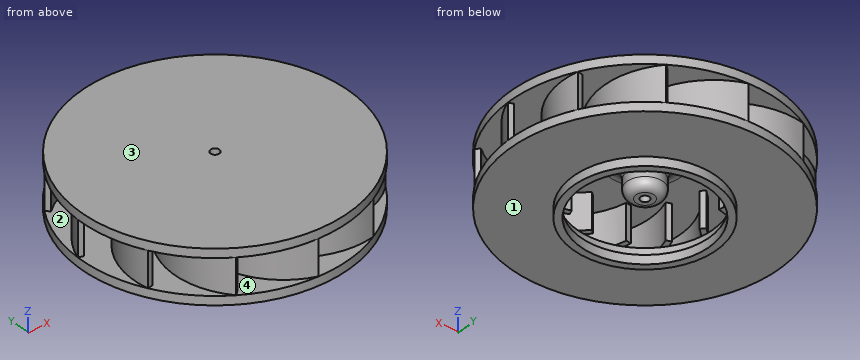
```python
from build123d import *

# Parameters (mm, degrees)
SKETCH_1_R          = 15
EXTRUDE_1_DEPTH     = 1
EXTRUDE_4_DEPTH     = 5
SKETCH_3_R          = 2
EXTRUDE_2_DEPTH     = 4
FILLET_1_R          = 2
FILLET_2_R          = 1
SKETCH_4_R          = 0.5
CUT_EXTRUDE_1_DEPTH = 5
SKETCH_5_R          = 15
EXTRUDE_3_DEPTH     = 1
SKETCH_6_R          = 8
SKETCH_6_R_2        = 7.2
EXTRUDE_4_2_DEPTH   = 1
SKETCH_7_R          = 7.6
CUT_EXTRUDE_2_DEPTH = 1


with BuildPart() as part:
    # 草图1 → 凸台-拉伸1 (new body)
    with BuildSketch(Plane.XY):
        Circle(SKETCH_1_R)
    extrude(amount=EXTRUDE_1_DEPTH)

    # 草图2 → Extrude 4 (add)
    with BuildSketch(Plane(origin=(0, 0, 0), x_dir=(-1, 0, 0), z_dir=(0, 0, -1))):
        with BuildLine():
            ThreePointArc((0, 7), (6.025450773, 10.246079868), (12.557822256, 8.203724775))
            Line((12.557822256, 8.203724775), (12.170554132, 7.745441675))
            ThreePointArc((12.170554132, 7.745441675), (6.082701111, 9.648817447), (0.467273577, 6.623628635))
            Line((0.467273577, 6.623628635), (0, 7))
        make_face()
        with BuildLine():
            ThreePointArc((3.5, 6.062177826), (10.341233372, 5.860640068), (14.977255477, 0.825722933))
            Line((14.977255477, 0.825722933), (14.412729894, 0.622472188))
            ThreePointArc((14.412729894, 0.622472188), (10.092182409, 5.31477047), (3.716485105, 5.502593875))
            Line((3.716485105, 5.502593875), (3.5, 6.062177826))
        make_face()
        with BuildLine():
            ThreePointArc((6.062177826, 3.5), (11.886090841, -0.095153505), (13.383545189, -6.773530702))
            Line((13.383545189, -6.773530702), (12.79302632, -6.667288219))
            ThreePointArc((12.79302632, -6.667288219), (11.397471581, -0.443364962), (5.969867451, 2.907143529))
            Line((5.969867451, 2.907143529), (6.062177826, 3.5))
        make_face()
        with BuildLine():
            ThreePointArc((7, 0), (10.246079868, -6.025450773), (8.203724775, -12.557822256))
            Line((8.203724775, -12.557822256), (7.745441675, -12.170554132))
            ThreePointArc((7.745441675, -12.170554132), (9.648817447, -6.082701111), (6.623628635, -0.467273577))
            Line((6.623628635, -0.467273577), (7, 0))
        make_face()
        with BuildLine():
            ThreePointArc((6.062177826, -3.5), (5.860640068, -10.341233372), (0.825722933, -14.977255477))
            Line((0.825722933, -14.977255477), (0.622472188, -14.412729894))
            ThreePointArc((0.622472188, -14.412729894), (5.31477047, -10.092182409), (5.502593875, -3.716485105))
            Line((5.502593875, -3.716485105), (6.062177826, -3.5))
        make_face()
        with BuildLine():
            ThreePointArc((3.5, -6.062177826), (-0.095153505, -11.886090841), (-6.773530702, -13.383545189))
            Line((-6.773530702, -13.383545189), (-6.667288219, -12.79302632))
            ThreePointArc((-6.667288219, -12.79302632), (-0.443364962, -11.397471581), (2.907143529, -5.969867451))
            Line((2.907143529, -5.969867451), (3.5, -6.062177826))
        make_face()
        with BuildLine():
            ThreePointArc((0, -7), (-6.025450773, -10.246079868), (-12.557822256, -8.203724775))
            Line((-12.557822256, -8.203724775), (-12.170554132, -7.745441675))
            ThreePointArc((-12.170554132, -7.745441675), (-6.082701111, -9.648817447), (-0.467273577, -6.623628635))
            Line((-0.467273577, -6.623628635), (0, -7))
        make_face()
        with BuildLine():
            ThreePointArc((-3.5, -6.062177826), (-10.341233372, -5.860640068), (-14.977255477, -0.825722933))
            Line((-14.977255477, -0.825722933), (-14.412729894, -0.622472188))
            ThreePointArc((-14.412729894, -0.622472188), (-10.092182409, -5.31477047), (-3.716485105, -5.502593875))
            Line((-3.716485105, -5.502593875), (-3.5, -6.062177826))
        make_face()
        with BuildLine():
            ThreePointArc((-6.062177826, -3.5), (-11.886090841, 0.095153505), (-13.383545189, 6.773530702))
            Line((-13.383545189, 6.773530702), (-12.79302632, 6.667288219))
            ThreePointArc((-12.79302632, 6.667288219), (-11.397471581, 0.443364962), (-5.969867451, -2.907143529))
            Line((-5.969867451, -2.907143529), (-6.062177826, -3.5))
        make_face()
        with BuildLine():
            ThreePointArc((-7, 0), (-10.246079868, 6.025450773), (-8.203724775, 12.557822256))
            Line((-8.203724775, 12.557822256), (-7.745441675, 12.170554132))
            ThreePointArc((-7.745441675, 12.170554132), (-9.648817447, 6.082701111), (-6.623628635, 0.467273577))
            Line((-6.623628635, 0.467273577), (-7, 0))
        make_face()
        with BuildLine():
            ThreePointArc((-6.062177826, 3.5), (-5.860640068, 10.341233372), (-0.825722933, 14.977255477))
            Line((-0.825722933, 14.977255477), (-0.622472188, 14.412729894))
            ThreePointArc((-0.622472188, 14.412729894), (-5.31477047, 10.092182409), (-5.502593875, 3.716485105))
            Line((-5.502593875, 3.716485105), (-6.062177826, 3.5))
        make_face()
        with BuildLine():
            ThreePointArc((-3.5, 6.062177826), (0.095153505, 11.886090841), (6.773530702, 13.383545189))
            Line((6.773530702, 13.383545189), (6.667288219, 12.79302632))
            ThreePointArc((6.667288219, 12.79302632), (0.443364962, 11.397471581), (-2.907143529, 5.969867451))
            Line((-2.907143529, 5.969867451), (-3.5, 6.062177826))
        make_face()
    extrude(amount=EXTRUDE_4_DEPTH)

    # 草图3 → 凸台-拉伸2 (add)
    with BuildSketch(Plane(origin=(0, 0, 0), x_dir=(-1, 0, 0), z_dir=(0, 0, -1))):
        with Locations(Location((0, 0, 0), (0, 0, 180))):
            Circle(SKETCH_3_R)
    extrude(amount=EXTRUDE_2_DEPTH)

    # 圆角1
    fillet_1_edges = [part.edges().sort_by_distance(p)[0] for p in [
        (-2, 0, 0),
    ]]
    fillet(fillet_1_edges, radius=FILLET_1_R)

    # 圆角2
    fillet_2_edges = [part.edges().sort_by_distance(p)[0] for p in [
        (-2, 0, -4),
    ]]
    fillet(fillet_2_edges, radius=FILLET_2_R)

    # 草图4 → 切除-拉伸1 (cut)
    with BuildSketch(Plane.XY.offset(1)):
        Circle(SKETCH_4_R)
    extrude(amount=-CUT_EXTRUDE_1_DEPTH, mode=Mode.SUBTRACT)

    # 草图5 → 凸台-拉伸3 (add)
    with BuildSketch(Plane(origin=(0, 0, -5), x_dir=(-1, 0, 0), z_dir=(0, 0, -1))):
        with Locations(Location((0, 0, 0), (0, 0, 3.155624395))):
            Circle(SKETCH_5_R)
    extrude(amount=-EXTRUDE_3_DEPTH)

    # 草图6 → Extrude 4 2 (add)
    with BuildSketch(Plane(origin=(0, 0, -5), x_dir=(-1, 0, 0), z_dir=(0, 0, -1))):
        Circle(SKETCH_6_R)
        Circle(SKETCH_6_R_2, mode=Mode.SUBTRACT)
    extrude(amount=EXTRUDE_4_2_DEPTH)

    # 草图7 → 切除-拉伸2 (cut)
    with BuildSketch(Plane(origin=(0, 0, -5), x_dir=(-1, 0, 0), z_dir=(0, 0, -1))):
        Circle(SKETCH_7_R)
    extrude(amount=-CUT_EXTRUDE_2_DEPTH, mode=Mode.SUBTRACT)


solid = part.part
```
Source: CAD feature listing. Evaluate the final solid. Frame: model axes, mm. Face numbers are marked on the shaded views. A direction names the side the tool comes from. Coordinates: 2 decimals unless noted, no trailing zeros. Order: outer loops, then holes, each group sorted by start corner. A loop starts at its lowest first (then second) coordinate and runs counter-clockwise, first axis right, second up. Notation, with made-up numbers: (83.5, 89.25) - (118.5, 89.25) arc R8 ccw to (118.5, 98.25) - close; hole circle Ø1 at (-0.75, 3). An arc over 180 degrees is marked (long way). One line per item, written item: value.
1) Cut plane A-A on y = -8.75. Output: boundary loops of the cut face in (x, z), plus the area to 3 significant figures.
Computed values:
outline: (-12.18, -5) - (12.18, -5) - (12.18, -4) - (11.84, -4) - (11.84, 0) - (12.18, 0) - (12.18, 1) - (-12.18, 1) - (-12.18, 0) - (-10.08, 0) - (-10.08, -4) - (-12.18, -4) - close; hole (-9.47, -4) - (-6.41, -4) - (-6.41, 0) - (-9.47, 0) - close; hole (-5.79, -4) - (-2.62, -4) - (-2.62, 0) - (-5.79, 0) - close; hole (-1.94, -4) - (1.89, -4) - (1.89, 0) - (-1.94, 0) - close; hole (3.06, -4) - (10.68, -4) - (10.68, 0) - (3.06, 0) - close
area: 65.7 mm^2
2) Reachability of the marked faces 3 and 4 from +Z, -Z, +X, -X, +Y, -Y: full face, straight path, thin tool, end or side. Return the list, or none.
Computed values:
face 3: +Z, +X, -X, +Y, -Y
face 4: none
3) Ray query, line 1 (Y direction, x = -0.25, z = -4.5); line 2 (Z direction, x = 4.25, y = 13.75); line 3 (Y direction, x = 10.5, z = -3). Return the intervals inside material, ascending. Write a range as [from, to].
Computed values:
line 1: y = [-15, -7.6], [7.6, 15]
line 2: z = [-5, -4], [0, 1]
line 3: y = [-9.5, -8.84], [-5.79, -5.11], [-1.43, -0.61]
4) Cut plane B-B on z = -0.5. State how many separate pieces and enclosed holes the cut face has, plus the area to 3 significant figures.
Computed values:
separate pieces: 13
enclosed holes: 1
area: 120 mm^2
5) Mould query, pull axis X, two halves, no side actions, for the marked faces 1 and 2. Classes: released by +X, released by -X, zero draft, split by the parting line, or undercut.
Computed values:
face 1: zero draft
face 2: undercut
6) Contact query for flat-ended pins moving along their axis: pin 1 (1.5 mm diameter, centred on y = 6.5, z = -2, fed in from -X); pin 2 (5 mm diameter, centred on x = 3.5, y = -5.5, fed in from -Z); pin 3 (3 mm diameter, centred on y = 9, z = -5, fed in from -X); pin 4 (8 mm diameter, centred on x = 11, y = 8, fed in from -Z). Output: stop coordinate, or through.
Computed values:
pin 1: stops at x = -10.57
pin 2: stops at z = -6
pin 3: stops at x = -12.99
pin 4: stops at z = -5
